Input: part model. Units: mm. Frame: model coordinates. Face numbers are marked on the shaded views. Round coordinates to 2 decimals unless told otherwise and drop trailing zeros. Loops run counter-clockwise (first coordinate to the right, second up) from the corner with the lowest first, then second, coordinate; pieces in that order, holes last. Notation, with made-up numbers: (-28, 7.25) - (-6, 7.25) arc R20 cw to (-6, 11.25) - close; hole circle Ø4 at (30.5, 54). An arc over 180 degrees is marked (long way). Write each question's results on one line, items separated by ' | '.
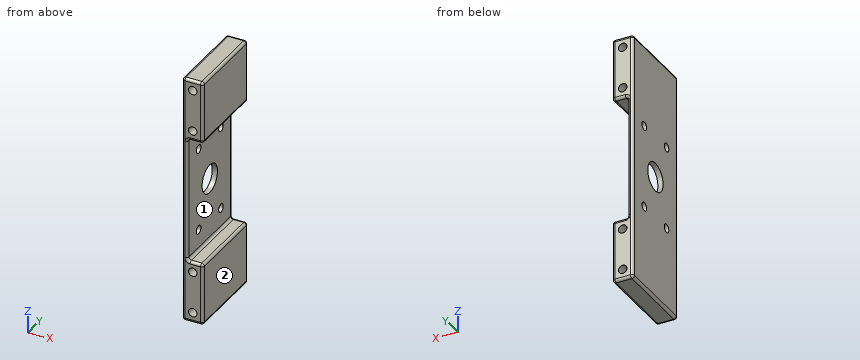
Autodesk Inventor part; units mm, degrees
ref_plane "YZ Plane" through (0, 0, 0) normal (1, 0, 0) x (0, 1, 0)
ref_plane "XZ Plane" through (0, 0, 0) normal (0, 1, 0) x (-1, 0, 0)
ref_plane "XY Plane" through (0, 0, 0) normal (0, 0, 1) x (1, 0, 0)
sketch "Sketch1" plane through (0, 0, 0) normal (0, 1, 0) x (-1, 0, 0)
  line L0 (0, 0) -> (-3.175, 0)
  line L1 (-3.175, 0) -> (-3.175, 101.6)
  line L2 (-3.175, 101.6) -> (0, 101.6)
  line L3 (0, 101.6) -> (0, 0)
  line L4 (0, 0) -> (-3.175, 0)
  line L5 (-3.175, 0) -> (-3.175, -25.4)
  line L6 (-3.175, -25.4) -> (0, -25.4)
  line L7 (0, -25.4) -> (0, 0)
  line L8 (0, 101.6) -> (-3.175, 101.6)
  line L9 (-3.175, 101.6) -> (-3.175, 127)
  line L10 (-3.175, 127) -> (0, 127)
  line L11 (0, 127) -> (0, 101.6)
  circle A0 centre (-6.35, 120.65) radius 2.5797
  circle A1 centre (-6.35, 95.25) radius 2.5797
  line L12 (0, 127) -> (-12.7, 127)
  line L13 (-12.7, 127) -> (-12.7, 88.9)
  line L14 (-12.7, 88.9) -> (0, 88.9)
  line L15 (0, 88.9) -> (0, 127)
  line L16 (25.4, 50.8) -> (-25.4, 50.8)
  line L17 (25.4, 50.8) -> (76.2, 50.8) construction
  line L18 (-3.175, 101.6) -> (-3.175, 0)
  line L19 (-3.175, 0) -> (0, 0)
  line L20 (0, 0) -> (0, 101.6)
  line L21 (0, 0) -> (-3.175, 0)
  line L22 (-3.175, 0) -> (-3.175, -25.4)
  line L23 (-3.175, -25.4) -> (0, -25.4)
  line L24 (0, -25.4) -> (0, 0)
  circle A2 centre (-6.35, -19.05) radius 2.5797
  circle A3 centre (-6.35, 6.35) radius 2.5797
  line L25 (0, -25.4) -> (-12.7, -25.4)
  line L26 (-12.7, -25.4) -> (-12.7, 12.7)
  line L27 (-12.7, 12.7) -> (0, 12.7)
  line L28 (0, 12.7) -> (0, -25.4)
  point P0 (-3.175, 88.9)
  point P1 (-3.175, 12.7)
  dimension "d25" = 3.175
  dimension "d26" = 101.6
  dimension "d27" = 3.175
  dimension "d28" = 25.4
  dimension "d29" = 3.175
  dimension "d30" = 25.4
  dimension "d31" = 0
  dimension "d32" = 25.4
  dimension "d33" = 6.35
  dimension "d34" = 5.1594
  dimension "d35" = 5.1594
  dimension "d36" = 12.7
  dimension "d37" = 38.1
  dimension "d38" = 6.35
  dimension "d39" = 50.8
  dimension "d40" = 180
  dimension "d41" = 50.8
  dimension "d42" = 25.4
extrude "Extrusion1" add sketch "Sketch1" along normal blind 50.8
sketch "Sketch3" plane through (3.175, 0, 88.9) normal (1, 0, 0) x (0, 0, -1)
  circle A0 centre (12.7, 12.7) radius 2.5797
  line L0 (0, 0) -> (76.2, 0)
  line L1 (0, 0) -> (0, 50.8)
  circle A1 centre (63.5, 12.7) radius 2.5797
  circle A2 centre (12.7, 38.1) radius 2.5797
  circle A3 centre (63.5, 38.1) radius 2.5797
  circle A4 centre (38.1, 25.4) radius 8.7312
  point P0 (88.9, 0)
  dimension "d43" = 12.7
  dimension "d44" = 12.7
  dimension "d45" = 5.1594
  dimension "d48" = 50.8
  dimension "d51" = 25.4
  dimension "d56" = 17.4625
  dimension "d57" = 25.4
  dimension "d58" = 38.1
extrude "Extrusion3" cut sketch "Sketch3" against normal blind 50.8
fillet "Fillet2" radius 1.5875 24 edges at (7.9375, 50.8, 88.9) (7.9375, 0, 88.9) (3.175, 25.4, 88.9) (12.7, 25.4, 88.9) (12.7, 25.4, 127) (12.7, 50.8, 107.95) (6.35, 50.8, 127) (0, 25.4, 127) (12.7, 0, 107.95) (6.35, 0, 127) (3.175, 50.8, 50.8) (3.175, 0, 50.8) (3.175, 25.4, 12.7) (7.9375, 50.8, 12.7) (7.9375, 0, 12.7) (12.7, 25.4, 12.7) (12.7, 50.8, -6.35) (12.7, 0, -6.35) (12.7, 25.4, -25.4) (6.35, 50.8, -25.4) (6.35, 0, -25.4) (0, 25.4, -25.4) (0, 0, 50.8) (0, 50.8, 50.8)
equation "\"d35\" = d34"
properties part number "Connector plate"
1. Contact query for a flat-ended pin moving along its axis: pin 1 (22.5 mm diameter, centred on y = 25.4, z = 50.8, fed in from +X) (3 decimals). Output: stop coordinate, or through.
Answer:
pin 1: x = 3.175
2. Section query D-D, the plane y = 8. Output: boundary loops of the cut face in (x, z) (3 decimals), plus the area to 3 significant figures.
Answer:
outline: (0, -23.813) arc R1.587 ccw to (1.587, -25.4) - (11.113, -25.4) arc R1.587 ccw to (12.7, -23.813) - (12.7, 11.113) arc R1.587 ccw to (11.113, 12.7) - (4.762, 12.7) arc R1.587 cw to (3.175, 14.287) - (3.175, 87.313) arc R1.587 cw to (4.762, 88.9) - (11.113, 88.9) arc R1.587 ccw to (12.7, 90.487) - (12.7, 125.413) arc R1.587 ccw to (11.113, 127) - (1.587, 127) arc R1.587 ccw to (0, 125.413) - close; hole circle Ø5.159 at (6.35, -19.05); hole circle Ø5.159 at (6.35, 6.35); hole circle Ø5.159 at (6.35, 95.25); hole circle Ø5.159 at (6.35, 120.65) | area: 1,120 mm^2
3. Mould query, pull axis Z, two halves, no side actions, for the marked faces 1 and 2. Classes: pulls with the +Z half, pulls with the -Z half, needs draft (parallel to the pull), parting line crosses it, or undercut.
Answer:
face 1: undercut | face 2: needs draft
4. Section query C-C, the plane z = 76.2. Count the separate pieces of the cut face and the enclosed holes in it, plus the area to 3 significant figures.
Answer:
separate pieces: 3 | enclosed holes: 0 | area: 126 mm^2
5. Line query: line 1 (Z direction, x = 6.35, y = 35.5); line 2 (Z direction, x = 4.75, y = 23); line 3 (Z direction, x = 10.5, y = 48.5). Output: solid intervals per line, ascending. Write a range as [from, to].
Answer:
line 1: [-25.4, -21.63], [-16.47, 3.77], [8.93, 12.7], [88.9, 92.67], [97.83, 118.07], [123.23, 127] | line 2: [-25.4, -21.07], [-17.03, 4.33], [8.37, 12.7], [88.9, 93.23], [97.27, 118.63], [122.67, 127] | line 3: [-25.4, 12.7], [88.9, 127]
6. Section query A-A, the plane y = 38.1. Output: boundary loops of the cut face in (x, z) (3 decimals).
Answer:
outline: (0, -23.813) arc R1.587 ccw to (1.587, -25.4) - (11.113, -25.4) arc R1.587 ccw to (12.7, -23.813) - (12.7, 11.113) arc R1.587 ccw to (11.113, 12.7) - (4.762, 12.7) arc R1.587 cw to (3.175, 14.287) - (3.175, 22.82) - (0, 22.82) - close; (0, 27.98) - (3.175, 27.98) - (3.175, 73.62) - (0, 73.62) - close; (0, 78.78) - (3.175, 78.78) - (3.175, 87.313) arc R1.587 cw to (4.762, 88.9) - (11.113, 88.9) arc R1.587 ccw to (12.7, 90.487) - (12.7, 125.413) arc R1.587 ccw to (11.113, 127) - (1.587, 127) arc R1.587 ccw to (0, 125.413) - close; hole circle Ø5.159 at (6.35, -19.05); hole circle Ø5.159 at (6.35, 6.35); hole circle Ø5.159 at (6.35, 95.25); hole circle Ø5.159 at (6.35, 120.65)
7. Section query B-B, the plane z = 95.25. Output: boundary loops of the cut face in (x, y).
Answer:
outline: (0, 1.59) arc R1.59 ccw to (1.59, 0) - (3.77, 0) - (3.77, 50.8) - (1.59, 50.8) arc R1.59 ccw to (0, 49.21) - close; (8.93, 0) - (11.11, 0) arc R1.59 ccw to (12.7, 1.59) - (12.7, 49.21) arc R1.59 ccw to (11.11, 50.8) - (8.93, 50.8) - close
